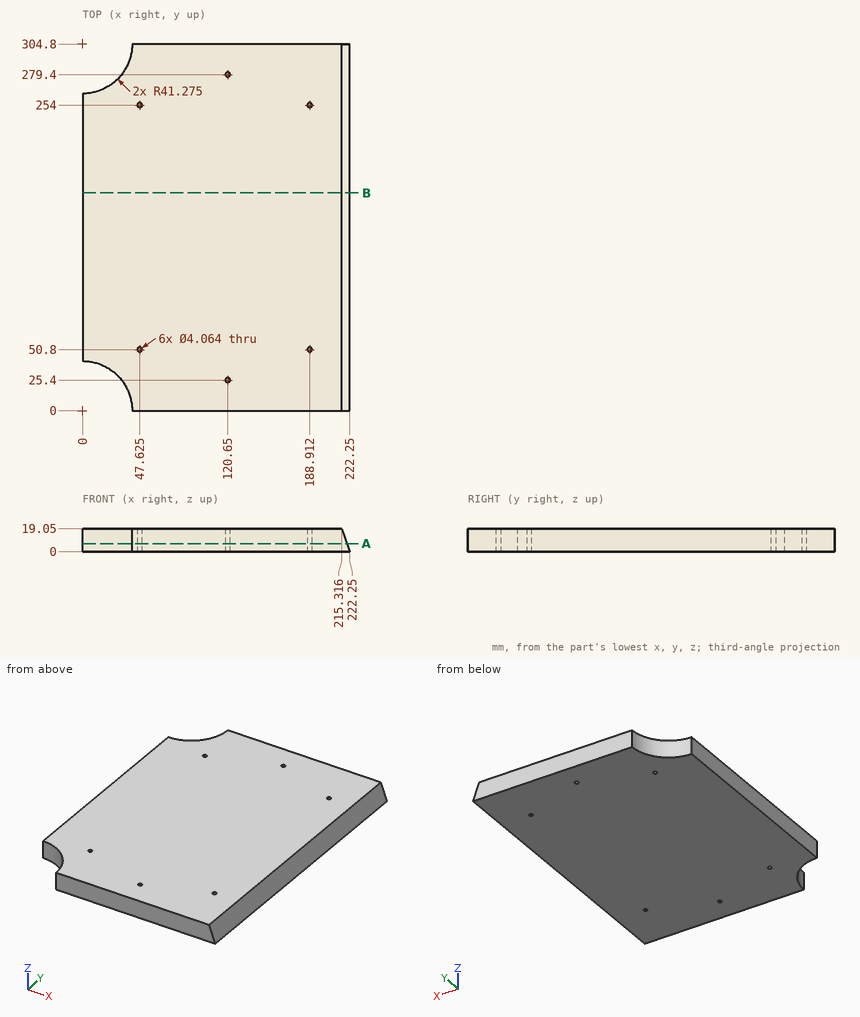
Design review of the part shown in the three views and the two pictorial views. Dimensions are in mm from the part's minimum x, y and z. Coordinates: 2 decimals unless noted, no trailing zeros. Write each loop counter-clockwise with the first axis right and the second up, starting at its lowest first coordinate (ties: lowest second). Pieces come first, ordered by that corner, then holes.
1) We need section B-B on y = 181. State the section outline as (x, z) points.
2) To check wall thickness, follow probe 1 along Y at (x, z) = (120.65, 7); probe 2 along X at (y, z) = (254.5, 2.5) (1 decimal); probe 3 along X at (y, z) = (254, 9) (1 decimal). State the ranges of each line that lie inside material, in increasing order.
3) We need section A-A on z = 6.5. Count the separate pieces of the cut face and the enclosed holes in it, then the cut area to 3 significant figures.
4) Clearance check with flat-ended pins moving along their axes: pin 1 Ø2.5 at (x, y) = (188.91, 50.8) entering from +Z; pin 2 Ø10 at (y, z) = (157, 15) entering from +X. State where each tip first meets the part, or that it passes through.
Answer list:
1. outline: (0, 0) - (222.25, 0) - (215.32, 19.05) - (0, 19.05) - close
2. probe 1: y = 0 to 23.37, 27.43 to 277.37, 281.43 to 304.8
2. probe 2: x = 0 to 45.7, 49.6 to 186.9, 190.9 to 221.3
2. probe 3: x = 0 to 45.6, 49.7 to 186.9, 190.9 to 219
3. separate pieces: 1
3. enclosed holes: 6
3. area: 64,300 mm2
4. pin 1: passes through
4. pin 2: stops at x = 218.61
